Work out the finished part from the listing and answer in its coordinate system (mm). A direction names the side the tool comes from. Round coordinates to 2 decimals unless told otherwise and drop trailing zeros. Write each loop counter-clockwise with the first axis right and the second up, starting at its lowest first coordinate (ties: lowest second). Pieces come first, ordered by that corner, then holes. Notation, with made-up numbers: (76.25, 61) - (100.25, 61) arc R20 cw to (100.25, 79) - close; hole circle Ø9 at (-38.5, 1). An arc over 180 degrees is marked (long way). Answer as a JSON object with one key per item and string values.
```python
from build123d import *

# Parameters (mm, degrees)
BOX_W        = 30.95
BOX_H        = 30.95
BOX_DEPTH    = 4.6
BOX001_W     = 30.975
BOX001_H     = 24
BOX001_DEPTH = 0.5
BOX002_W     = 24
BOX002_H     = 30.975
BOX002_DEPTH = 0.5
BOX003_W     = 20.32
BOX003_H     = 27.4
BOX003_DEPTH = 4
CHAMFER_SIZE = 2
BOX004_W     = 2.5
BOX004_H     = 1.75
BOX004_DEPTH = 3
BOX005_W     = 27.4
BOX005_H     = 20.32
BOX005_DEPTH = 4
BOX006_W     = 5.1
BOX006_H     = 3.3
BOX006_DEPTH = 4
BOX007_W     = 3.4
BOX007_H     = 1.7
BOX007_DEPTH = 4.6
BOX008_W     = 3.4
BOX008_H     = 1.7
BOX008_DEPTH = 4.6
FILLET_R     = 1
FILLET001_R  = 1
FILLET002_R  = 1


with BuildPart() as part:
    # Box → Box (join)
    with BuildSketch(Plane(origin=(-15.475, -15.475, 0), x_dir=(1, 0, 0), z_dir=(0, 0, 1))):
        with Locations((15.475, 15.475)):
            Rectangle(BOX_W, BOX_H)
    extrude(amount=BOX_DEPTH)

    # Box001 → Box001 (cut)
    with BuildSketch(Plane(origin=(-15.475, -12, 0), x_dir=(1, 0, 0), z_dir=(0, 0, 1))):
        with Locations((15.4875, 12)):
            Rectangle(BOX001_W, BOX001_H)
    extrude(amount=BOX001_DEPTH, mode=Mode.SUBTRACT)

    # Box002 → Box002 (cut)
    with BuildSketch(Plane(origin=(-12, -15.475, 0), x_dir=(1, 0, 0), z_dir=(0, 0, 1))):
        with Locations((12, 15.4875)):
            Rectangle(BOX002_W, BOX002_H)
    extrude(amount=BOX002_DEPTH, mode=Mode.SUBTRACT)

    # Box003 → Box003 (cut)
    with BuildSketch(Plane(origin=(-10.252, -13.7, 0.6), x_dir=(1, 0, 0), z_dir=(0, 0, 1))):
        with Locations((10.16, 13.7)):
            Rectangle(BOX003_W, BOX003_H)
    extrude(amount=BOX003_DEPTH, mode=Mode.SUBTRACT)

    # Chamfer
    chamfer_edges = [part.edges().sort_by_distance(p)[0] for p in [
        (-15.475, 15.475, 2.3),
    ]]
    chamfer(chamfer_edges, length=CHAMFER_SIZE)

    # Box004 → Box004 (cut)
    with BuildSketch(Plane(origin=(-13.625, 11.8, 2.5), x_dir=(0.707107, 0.707107, 0), z_dir=(0, 0, 1))):
        with Locations((1.25, 0.875)):
            Rectangle(BOX004_W, BOX004_H)
    extrude(amount=BOX004_DEPTH, mode=Mode.SUBTRACT)

    # Box005 → Box005 (cut)
    with BuildSketch(Plane(origin=(-13.75, -10.3, 0.6), x_dir=(1, 0, 0), z_dir=(0, 0, 1))):
        with Locations((13.7, 10.16)):
            Rectangle(BOX005_W, BOX005_H)
    extrude(amount=BOX005_DEPTH, mode=Mode.SUBTRACT)

    # Box006 → Box006 (cut)
    with BuildSketch(Plane(origin=(-11.45, 7.75, 0.6), x_dir=(0.707107, 0.707107, 0), z_dir=(0, 0, 1))):
        with Locations((2.55, 1.65)):
            Rectangle(BOX006_W, BOX006_H)
    extrude(amount=BOX006_DEPTH, mode=Mode.SUBTRACT)

    # Box007 → Box007 (cut)
    with BuildSketch(Plane(origin=(-12.875, -14, 0), x_dir=(0.707107, 0.707107, 0), z_dir=(0, 0, 1))):
        with Locations((1.7, 0.85)):
            Rectangle(BOX007_W, BOX007_H)
    extrude(amount=BOX007_DEPTH, mode=Mode.SUBTRACT)

    # Box008 → Box008 (cut)
    with BuildSketch(Plane(origin=(10.875, 10, 0), x_dir=(0.707107, 0.707107, 0), z_dir=(0, 0, 1))):
        with Locations((1.7, 0.85)):
            Rectangle(BOX008_W, BOX008_H)
    extrude(amount=BOX008_DEPTH, mode=Mode.SUBTRACT)

    # Fillet
    fillet_edges = [part.edges().sort_by_distance(p)[0] for p in [
        (-15.475, -15.475, 2.3),
    ]]
    fillet(fillet_edges, radius=FILLET_R)

    # Fillet001
    fillet001_edges = [part.edges().sort_by_distance(p)[0] for p in [
        (15.475, -15.475, 2.3),
    ]]
    fillet(fillet001_edges, radius=FILLET001_R)

    # Fillet002
    fillet002_edges = [part.edges().sort_by_distance(p)[0] for p in [
        (15.475, 15.475, 2.3),
    ]]
    fillet(fillet002_edges, radius=FILLET002_R)


solid = part.part
```
Item 1: Each of these flat-tipped pins is pushed along its axis until it touches: P1, Ø10, axis at x = -5.5, y = -11.5, coming from the +Z side; P2, Ø8, axis at x = -2, y = 2, coming from the +Z side; P3, Ø2, axis at x = 0, y = 11, coming from the -Z side. Where does it stop, or does it pass through?
Results found:
{"P1": "z = 4.6", "P2": "z = 0.6", "P3": "z = 0.5"}
Item 2: Determine the mould class of faces 1 (the flat face through (0, 15.475, 2)), 2 (the flat face through (10.068, -12, 3)), 3 (the cylindrical face through (15.19, 15.174, 2.332)) for opening direction X: pulls with the +X half, pulls with the -X half, needs draft (parallel to the pull), parting line crosses it, or undercut.
Results found:
{"face 1": "needs draft", "face 2": "undercut", "face 3": "pulls with the +X half"}
Item 3: A cutting plane is placed at C-C (x = -12.5). Write down the section's boundary in (y, z) (3 decimals).
Results found:
{"outline": "(-15.475, 0) - (-13.625, 0) - (-13.625, 4.6) - (-15.475, 4.6) - close; (-11.221, 0.5) - (12, 0.5) - (12, 0) - (15.475, 0) - (15.475, 4.6) - (14.211, 4.6) - (14.211, 2.5) - (12.925, 2.5) - (12.925, 4.6) - (11.367, 4.6) - (11.367, 0.6) - (-10.3, 0.6) - (-10.3, 4.6) - (-11.221, 4.6) - close"}
Item 4: For faces 4 (the flat face through (15.475, 0, 2)), 5 (the flat face through (-12.89, -11.61, 2.27)), 6 (the flat face through (-12, -10.3, 3)), determine the directions among +Z, -Z, +X, -X, +Y, -Y from which every point of the face is accessible in a straight line to the end or side of a thin tool.
Results found:
{"face 4": "+Z, -Z, +X, +Y, -Y", "face 5": "+Z, -Z", "face 6": "+Z"}
Item 5: A cutting plane is placed at A-A (z = 1.85). Give the number of separate pieces and of enclosed holes in the cut face, and give its area (3 significant figures).
Results found:
{"separate pieces": "2", "enclosed holes": "2", "area": "237 mm²"}
Item 6: A cutting plane is placed at B-B (y = -6). Write down the section's boundary in (x, z) (3 decimals).
Results found:
{"outline": "(-15.475, 0.5) - (15.475, 0.5) - (15.475, 4.6) - (13.65, 4.6) - (13.65, 0.6) - (-13.75, 0.6) - (-13.75, 4.6) - (-15.475, 4.6) - close"}
Item 7: Consider line 1 along Y through (x, z) = (8, 1.15) (3 decimals); line 2 along X through (y, z) = (-2, 4.4) (3 decimals); line 3 along Y through (x, z) = (-11.5, 4) (3 decimals). Determine where each line is inside the solid, lowest interval first.
Results found:
{"line 1": "-15.475 to -13.7, 13.7 to 15.475", "line 2": "-15.475 to -13.75, 13.65 to 15.475", "line 3": "-15.475 to -12.625, -10.567 to -10.3, 12.367 to 15.475"}
